Autodesk Fusion 360 part; units mm, degrees
sketch "Sketch1" plane through (0, 0, 0) normal (0, 1, 0) x (1, 0, 0)
  line L0 (25, -25) -> (152.63, -25)
  line L1 (152.63, -25) -> (152.63, -110.47)
  line L2 (152.63, -110.47) -> (25, -110.47)
  line L3 (25, -110.47) -> (25, -25)
  line L4 (25, -67.735) -> (152.63, -67.735) construction
  line L5 (88.815, -25) -> (88.815, -110.47) construction
  line L6 (88.815, -67.735) -> (25, -67.735) construction
  line L7 (56.9075, -67.735) -> (56.9075, -25) construction
  line L8 (56.9075, -67.735) -> (56.9075, -46.3675) construction
  line L9 (88.815, -67.735) -> (152.63, -67.735) construction
  line L10 (88.815, -67.735) -> (120.7225, -67.735) construction
  line L11 (120.7225, -67.735) -> (120.7225, -25) construction
  line L12 (120.7225, -67.735) -> (120.7225, -46.3675) construction
  circle A0 centre (56.9075, -46.3675) radius 20
  circle A1 centre (120.7225, -46.3675) radius 20
  line L13 (56.9075, -67.735) -> (56.9075, -110.47) construction
  line L14 (56.9075, -67.735) -> (56.9075, -89.1025) construction
  circle A2 centre (56.9075, -89.1025) radius 20
  line L15 (120.7225, -67.735) -> (120.7225, -110.47) construction
  line L16 (120.7225, -110.47) -> (120.7225, -89.1025) construction
  circle A3 centre (120.7225, -89.1025) radius 20
  line L17 (120.7225, -46.3675) -> (150.7225, -46.3675) construction
  line L18 (150.7225, -46.3675) -> (150.7225, -41.3675) construction
  line L19 (150.7225, -41.3675) -> (90.7225, -41.3675)
  line L20 (90.7225, -41.3675) -> (90.7225, -51.3675)
  line L21 (90.7225, -51.3675) -> (150.7225, -51.3675)
  line L22 (150.7225, -51.3675) -> (150.7225, -41.3675)
  line L23 (56.9075, -46.3675) -> (86.9075, -46.3675) construction
  line L24 (86.9075, -46.3675) -> (86.9075, -41.3675) construction
  line L25 (86.9075, -41.3675) -> (26.9075, -41.3675)
  line L26 (26.9075, -41.3675) -> (26.9075, -51.3675)
  line L27 (26.9075, -51.3675) -> (86.9075, -51.3675)
  line L28 (86.9075, -51.3675) -> (86.9075, -41.3675)
  line L29 (56.9075, -89.1025) -> (86.9075, -89.1025) construction
  line L30 (86.9075, -89.1025) -> (86.9075, -84.1025) construction
  line L31 (86.9075, -84.1025) -> (26.9075, -84.1025)
  line L32 (26.9075, -84.1025) -> (26.9075, -94.1025)
  line L33 (26.9075, -94.1025) -> (86.9075, -94.1025)
  line L34 (86.9075, -94.1025) -> (86.9075, -84.1025)
  line L35 (120.7225, -89.1025) -> (150.7225, -89.1025) construction
  line L36 (150.7225, -89.1025) -> (150.7225, -84.1025) construction
  line L37 (150.7225, -84.1025) -> (90.7225, -84.1025)
  line L38 (90.7225, -84.1025) -> (90.7225, -94.1025)
  line L39 (90.7225, -94.1025) -> (150.7225, -94.1025)
  line L40 (150.7225, -94.1025) -> (150.7225, -84.1025)
  dimension "d1" = 127.63
  dimension "d2" = 85.47
  dimension "d3" = 40
  dimension "d4" = 40
  dimension "d5" = 40
  dimension "d6" = 40
  dimension "d7" = 30
  dimension "d8" = 5
  dimension "d9" = 60
  dimension "d10" = 10
  dimension "d11" = 30
  dimension "d12" = 5
  dimension "d13" = 60
  dimension "d14" = 10
  dimension "d15" = 30
  dimension "d16" = 5
  dimension "d17" = 60
  dimension "d18" = 10
  dimension "d19" = 30
  dimension "d20" = 5
  dimension "d21" = 60
  dimension "d22" = 10
extrude "Extrude1" add sketch "Sketch1" against normal blind 20.19 contours L0 L1 L2 L3 | A0 L25 L27 | A0 L25 L27 L28 | A0 L25 | A0 L27 | A0 L25 L26 L27 | A1 L19 L21 | A1 L19 L21 L22 | A1 L19 | A1 L21 | A1 L19 L20 L21 | A2 L31 L33 | A2 L31 L33 L34 | A2 L31 | A2 L33 | A2 L31 L32 L33 | A3 L37 L39 | A3 L37 L39 L40 | A3 L37 | A3 L39 | A3 L37 L38 L39
extrude "Extrude2" cut sketch "Sketch1" against normal blind 11.43 contours A0 L25 L27 | A0 L25 L27 L28 | A0 L25 | A0 L27 | A0 L25 L26 L27 | A1 L19 L21 | A1 L19 L21 L22 | A1 L19 | A1 L21 | A1 L19 L20 L21 | A2 L31 L33 | A2 L31 L33 L34 | A2 L31 | A2 L33 | A2 L31 L32 L33 | A3 L37 L39 | A3 L37 L39 L40 | A3 L37 | A3 L39
extrude "Extrude3" cut sketch "Sketch1" against normal blind 11.43 contours A3 L37 L38 L39
extrude "Extrude4" cut 1 faces at (67.5433, -20.19, 53.49) along direction (0, 1, 0) blind 7
The listing builds one solid part. Answer for the finished solid, in the listing's coordinates (mm). Round coordinates to 2 decimals unless told otherwise and drop trailing zeros. Order: outer loops, then holes, each group sorted by start corner. A loop starts at its lowest first (then second) coordinate and runs counter-clockwise, first axis right, second up. Notation, with made-up numbers: (2.5, -26.5) -> (32.5, -26.5) arc R24 ccw to (32.5, -0.5) -> close; hole circle Ø2 at (63.5, -22.75). An arc over 180 degrees is marked (long way). Answer as CSV lines item,"result". Start each with the question number.
(1) For a pull along X with two mould halves and no side action, classify faces 1 (the face through (96, -6, 94.102)), 2 (the face through (88, -13.19, 67)) as +X half, -X half, draft (parallel to the pull), parting line (faces both ways), or undercut.
(2) The part is cut by section C-C (y = -8.75). Count the separate pieces of the cut face and the enclosed holes in it, then the cut area to 3 significant figures.
(3) Find the intervals of material crossed by probe 1 along Z at (x, y) = (31.5, -0.5); probe 2 along X at (y, z) = (-4.25, 89.5); probe 3 along X at (y, z) = (-11, 57), in increasing order. Write a range as from..to.
(4) The part is cut by section B-B (x = 49.5). Determine the outline of the cut face in (y, z).
(5) The part is cut by section A-A (z = 91.5). Determine the outline of the cut face in (x, y).
Evaluation:
1,face 1,"undercut"
1,face 2,"draft"
2,separate pieces,"1"
2,enclosed holes,"4"
2,area,"5,070 mm²"
3,probe 1,"25..41.37, 51.37..84.1, 94.1..110.47"
3,probe 2,"25..26.91, 86.91..90.72, 150.72..152.63"
3,probe 3,"25..39.97, 73.85..103.78, 137.66..152.63"
4,outline,"(-13.19, 25) -> (0, 25) -> (0, 27.79) -> (-11.43, 27.79) -> (-11.43, 64.95) -> (0, 64.95) -> (0, 70.52) -> (-11.43, 70.52) -> (-11.43, 107.68) -> (0, 107.68) -> (0, 110.47) -> (-13.19, 110.47) -> close"
5,outline,"(25, -13.19) -> (152.63, -13.19) -> (152.63, 0) -> (150.72, 0) -> (150.72, -11.43) -> (90.72, -11.43) -> (90.72, 0) -> (86.91, 0) -> (86.91, -11.43) -> (26.91, -11.43) -> (26.91, 0) -> (25, 0) -> close"
